```python
from build123d import *

# Parameters (mm, degrees)
SKETCH2_W             = 6.16625
SKETCH2_H             = 18.6
BOSS_EXTRUDE1_DEPTH   = 2
BOSS_EXTRUDE1_2_DEPTH = 2
SKETCH3_W             = 3
SKETCH3_H             = 48.6
BOSS_EXTRUDE2_DEPTH   = 13
FILLET1_R             = 1.25
CUT_EXTRUDE1_DEPTH    = 2
M3_CLEARANCE_HOLE1_D  = 3.6


with BuildPart() as part:
    # Sketch2 → Boss-Extrude1 (new body)
    with BuildSketch(Plane.XY.offset(11.211435671)):
        with Locations((-7.173848327, -28.012787822)):
            Rectangle(SKETCH2_W, SKETCH2_H)
    extrude(amount=BOSS_EXTRUDE1_DEPTH)



with BuildPart() as body_2:
    # Sketch2 → Boss-Extrude1 2 (new body)
    with BuildSketch(Plane.XY.offset(11.211435671)):
        with Locations((-7.173848327, -58.012787822)):
            Rectangle(SKETCH2_W, SKETCH2_H)
    extrude(amount=BOSS_EXTRUDE1_2_DEPTH)


with BuildPart() as part_1:
    add(part.part)

    add(body_2.part)  # Boss-Extrude2 merges body 2
    # Sketch3 → Boss-Extrude2 (add)
    with BuildSketch(Plane.XY.offset(13.211435671)):
        with Locations((-5.590723327, -43.012787822)):
            Rectangle(SKETCH3_W, SKETCH3_H)
    extrude(amount=BOSS_EXTRUDE2_DEPTH)

    # Fillet1
    fillet1_edges = [part_1.edges().sort_by_distance(p)[0] for p in [
        (-7.090723327, -58.012787822, 13.211435671),
        (-7.090723327, -28.012787822, 13.211435671),
    ]]
    fillet(fillet1_edges, radius=FILLET1_R)

    # Sketch4 → Cut-Extrude1 (cut)
    with BuildSketch(Plane(origin=(-7.090723327, 0, 0), x_dir=(0, 0, -1), z_dir=(1, 0, 0))):
        Polygon((-19.351262419, -29.850501062), (-22.101262419, -31.438214302), (-24.851262419, -29.850501062), (-24.851262419, -26.675074581), (-22.101262419, -25.087361341), (-19.351262419, -26.675074581), align=None)
        Polygon((-22.101262419, -60.938214302), (-19.351262419, -59.350501062), (-19.351262419, -56.175074581), (-22.101262419, -54.587361341), (-24.851262419, -56.175074581), (-24.851262419, -59.350501062), align=None)
    extrude(amount=CUT_EXTRUDE1_DEPTH, mode=Mode.SUBTRACT)

    # M3 Clearance Hole1 (through all)
    with Locations(Plane.ZY.offset(7.090723327)):
        with Locations((22.101262419, -57.762787822), (22.101262419, -28.262787822)):
            Hole(M3_CLEARANCE_HOLE1_D / 2)


solid = part_1.part
```
Design review of the part built by this model. Coordinates are the model's own, in mm. A direction names the side the tool comes from. Round coordinates to 2 decimals unless told otherwise and drop trailing zeros. Order: outer loops, then holes, each group sorted by start corner. A loop starts at its lowest first (then second) coordinate and runs counter-clockwise, first axis right, second up. Notation, with made-up numbers: (16, 58) - (36, 58) arc R8 ccw to (36, 65) - close; hole circle Ø8 at (50.25, 44.25). An arc over 180 degrees is marked (long way). One line per question, with ' | ' between items.
Item 1: Take a section at C-C, the plane z = 13.75. Write out the cut boundary in (x, y), then the cut area to 3 significant figures.
Checks:
outline: (-7.31, -67.31) - (-4.09, -67.31) - (-4.09, -18.71) - (-7.31, -18.71) - (-7.31, -37.31) - (-7.09, -37.31) - (-7.09, -48.71) - (-7.31, -48.71) - close | area: 154 mm²
Item 2: Draft analysis for pull direction Z (two halves, no side actions). For faces 4 (the face through (-6, -43, 26.211)), 5 (the face through (-6.105, -30.655, 23.457)), 6 (the face through (-6, -18.713, 17)), state which applies: +Z half, -Z half, draft (parallel to the pull), parting line (faces both ways), or undercut.
Checks:
face 4: +Z half | face 5: undercut | face 6: draft
Item 3: Take a section at D-D, the plane z = 16.5. Write out the cut boundary in (x, y).
Checks:
outline: (-7.09, -67.31) - (-4.09, -67.31) - (-4.09, -18.71) - (-7.09, -18.71) - close
Item 4: Take a section at B-B, the plane x = -5.75. Write out the cut boundary in (y, z).
Checks:
outline: (-67.31, 11.21) - (-48.71, 11.21) - (-48.71, 13.21) - (-37.31, 13.21) - (-37.31, 11.21) - (-18.71, 11.21) - (-18.71, 26.21) - (-67.31, 26.21) - close; hole (-60.94, 22.1) - (-59.35, 19.35) - (-56.18, 19.35) - (-54.59, 22.1) - (-56.18, 24.85) - (-59.35, 24.85) - close; hole (-31.44, 22.1) - (-29.85, 19.35) - (-26.68, 19.35) - (-25.09, 22.1) - (-26.68, 24.85) - (-29.85, 24.85) - close
Item 5: Machinability: for faces 1 (the face through (-6, -28, 24.851)), 2 (the face through (-4.091, -43, 19)), 3 (the face through (-9, -28, 13.211)), which of the approach directions +Z, -Z, +X, -X, +Y, -Y give a long, thin tool a straight path to every point of the face, cutting with its end or side? Answer none if there is none.
Checks:
face 1: -X | face 2: +Z, -Z, +X, +Y, -Y | face 3: +Z, -X, +Y, -Y
Item 6: For P1, Ø0.6, axis at x = -10, y = -58.5, coming from the +Z side; P2, Ø2, axis at y = -61.5, z = 23, coming from the -X side; P3, Ø2.5, axis at x = -5.5, y = -40.5, coming from the -Z side, all flat-tipped, find the tip position at first contact; note any pin that passes through.
Checks:
P1: z = 13.21 | P2: x = -7.09 | P3: z = 13.21
Item 7: Wall thickness on line 1 (Y direction, x = -4.75, z = 21); line 2 (Y direction, x = -7, z = 21.75); line 3 (X direction, y = -43, z = 25): over which ranges is each line inside the solid? List them lowest first. Write a range as [from, to].
Checks:
line 1: [-67.31, -59.19], [-56.34, -29.69], [-26.84, -18.71] | line 2: [-67.31, -60.74], [-54.79, -31.24], [-25.29, -18.71] | line 3: [-7.09, -4.09]
Item 8: Take a section at A-A, the plane y = -36.5. Write out the cut boundary in (x, z), then the cut area to 3 significant figures.
Checks:
outline: (-10.26, 11.21) - (-4.09, 11.21) - (-4.09, 26.21) - (-7.09, 26.21) - (-7.09, 14.46) arc R1.25 cw to (-8.34, 13.21) - (-10.26, 13.21) - close | area: 51.7 mm²
